from build123d import *

# Parameters (mm, degrees)
CBORE_FOR_M2_SHCS1_D           = 2.6
CBORE_FOR_M2_SHCS1_DEPTH       = 5
CBORE_FOR_M2_SHCS1_CBORE_D     = 4.4
CBORE_FOR_M2_SHCS1_CBORE_DEPTH = 2
CBORE_FOR_M2_SHCS1_TIP         = 0.781118805


with BuildPart() as part:
    # Sketch1 → Revolve1 (revolve)
    with BuildSketch(Plane.XY):
        Polygon((0, 0), (8, 0), (8, 3.5), (2, 3.5), (2, 14.5), (0, 14.5), align=None)
    revolve(axis=Axis((0, 14.5, 0), (0, -1, 0)))

    # CBORE for M2 SHCS1
    with Locations(Plane(origin=(-4.5, 3.5, 0), x_dir=(1, 0, 0), z_dir=(0, 1, 0))):
        with Locations((0, 0), (4.5, 4.5), (9, 0), (4.5, -4.5)):
            CounterBoreHole(CBORE_FOR_M2_SHCS1_D / 2, CBORE_FOR_M2_SHCS1_CBORE_D / 2, CBORE_FOR_M2_SHCS1_CBORE_DEPTH, depth=CBORE_FOR_M2_SHCS1_DEPTH)
            with Locations((0, 0, -(CBORE_FOR_M2_SHCS1_DEPTH + CBORE_FOR_M2_SHCS1_TIP / 2))):  # 118° drill point
                Cone(0, CBORE_FOR_M2_SHCS1_D / 2, CBORE_FOR_M2_SHCS1_TIP, mode=Mode.SUBTRACT)


solid = part.part
Geometry: final body of the model. Coordinates: model frame, mm. A direction names the side the tool comes from. Coordinates: 2 decimals unless noted, no trailing zeros. Order: outer loops, then holes, each group sorted by start corner. A loop starts at its lowest first (then second) coordinate and runs counter-clockwise, first axis right, second up.
1) Section B-B (x = -4.75). Return loops of the section in (y, z).
Result sheet:
outline: (0, -6.44) - (3.5, -6.44) - (3.5, -2.19) - (1.5, -2.19) - (1.5, -1.28) - (0, -1.28) - close; (0, 1.28) - (1.5, 1.28) - (1.5, 2.19) - (3.5, 2.19) - (3.5, 6.44) - (0, 6.44) - close
2) Draft query along Z for faces 1 (the cylindrical face through (0.28, 0.74, 5.77)), 2 (the cylindrical face through (-1.73, 1.77, -7.81)), 3 (the flat face through (2, 3.5, -2)). Return one class per face: released by +Z, released by -Z, zero draft, split by the parting line, or undercut.
Result sheet:
face 1: undercut
face 2: split by the parting line
face 3: zero draft
3) Ray query, probe 1 along Z at (x, y) = (0, 2.15); probe 2 along Z at (x, y) = (0, 0.6); probe 3 along Z at (x, y) = (4.5, 0.8). Return the intervals inside material, ascending.
Result sheet:
probe 1: z = -8 to -6.7, -2.3 to 2.3, 6.7 to 8
probe 2: z = -8 to -5.8, -3.2 to 3.2, 5.8 to 8
probe 3: z = -6.61 to -1.3, 1.3 to 6.61
4) Section A-A (z = 0). Return loops of the section in (x, y), then the cut area to 3 significant figures.
Result sheet:
outline: (-8, 0) - (-5.8, 0) - (-5.8, 1.5) - (-6.7, 1.5) - (-6.7, 3.5) - (-8, 3.5) - close; (-3.2, 0) - (3.2, 0) - (3.2, 1.5) - (2.3, 1.5) - (2.3, 3.5) - (2, 3.5) - (2, 14.5) - (-2, 14.5) - (-2, 3.5) - (-2.3, 3.5) - (-2.3, 1.5) - (-3.2, 1.5) - close; (5.8, 0) - (8, 0) - (8, 3.5) - (6.7, 3.5) - (6.7, 1.5) - (5.8, 1.5) - close
area: 74.6 mm2
5) First-contact query: P1, Ø4, axis at x = -4.5, z = 0, coming from the +Y side; P2, Ø2, axis at y = 7, z = -3.5, coming from the -X side; P3, Ø4, axis at y = 10.5, z = -3.5, coming from the +X side. Flat tips, straight axial feed; report the tip coordinate or a pass-through.
Result sheet:
P1: stops at y = 1.5
P2: passes through
P3: stops at x = 1.32
6) Set-up query: faces 4 (the cylindrical face through (0, 9, -2)), 5 (the flat face through (0, 14.5, 0)). Return all of +Z, -Z, +X, -X, +Y, -Y with unobstructed straight access to the full face (end or side cutting, diameter ignored); none if empty.
Result sheet:
face 4: +Y
face 5: +Z, -Z, +X, -X, +Y
7) Section C-C (x = 0). Return loops of the section in (y, z).
Result sheet:
outline: (0, -8) - (3.5, -8) - (3.5, -6.7) - (1.5, -6.7) - (1.5, -5.8) - (0, -5.8) - close; (0, -3.2) - (1.5, -3.2) - (1.5, -2.3) - (3.5, -2.3) - (3.5, -2) - (14.5, -2) - (14.5, 2) - (3.5, 2) - (3.5, 2.3) - (1.5, 2.3) - (1.5, 3.2) - (0, 3.2) - close; (0, 5.8) - (1.5, 5.8) - (1.5, 6.7) - (3.5, 6.7) - (3.5, 8) - (0, 8) - close
8) Section D-D (z = 4.75). Return loops of the section in (x, y), then the cut area to 3 significant figures.
Result sheet:
outline: (-6.44, 0) - (-1.28, 0) - (-1.28, 1.5) - (-2.19, 1.5) - (-2.19, 3.5) - (-6.44, 3.5) - close; (1.28, 0) - (6.44, 0) - (6.44, 3.5) - (2.19, 3.5) - (2.19, 1.5) - (1.28, 1.5) - close
area: 32.5 mm2
